Check sheet for the modelled part. Datum: model origin and axes. Units: mm. Face numbers are marked on the shaded views. A direction names the side the tool comes from. Coordinates: 2 decimals unless noted, no trailing zeros. Order: outer loops, then holes, each group sorted by start corner. A loop starts at its lowest first (then second) coordinate and runs counter-clockwise, first axis right, second up.
1. Thickness scan on line 1 (Y direction, x = 10, z = 2.3); line 2 (X direction, y = 20.5, z = 2.9); line 3 (X direction, y = 6.25, z = 2). Record the ranges inside material, lowest first.
2. Cross-section at C-C (x = 10). Enter the section's corners in (y, z) (3 decimals).
3. Set-up check for the marked faces 1 and 2: record each of +Z, -Z, +X, -X, +Y, -Y from which the full face is reachable in a straight line by a thin tool's end or side.
4. Cross-section at A-A (z = 2.8). Enter the section's corners in (x, y), then the cut area to 3 significant figures.
5. Cross-section at B-B (y = 20.5). Enter the section's corners in (x, z) (3 decimals).
6. Draft check along Y on the marked faces 3, 4, 5 and 6. Enter one of: released by +Y, released by -Y, zero draft, split by the parting line, or undercut.
Autodesk Inventor part; units mm, degrees
ref_plane "YZ Plane" through (0, 0, 0) normal (1, 0, 0) x (0, 1, 0)
ref_plane "XZ Plane" through (0, 0, 0) normal (0, 1, 0) x (-1, 0, 0)
ref_plane "XY Plane" through (0, 0, 0) normal (0, 0, 1) x (1, 0, 0)
sketch "Sketch1" plane through (0, 0, 0) normal (0, 0, 1) x (1, 0, 0)
  line L0 (0, 0) -> (20, 0)
  line L1 (20, 0) -> (20, 41)
  line L2 (20, 41) -> (0, 41)
  line L3 (0, 41) -> (0, 0)
  dimension "d0" = 20
  dimension "d1" = 41
extrude "Extrusion1" add sketch "Sketch1" along normal blind 4
sketch "Sketch2" plane through (0, 0, 4) normal (0, 0, 1) x (1, 0, 0)
  line L0 (20, 0) -> (20, 41)
  line L1 (20, 41) -> (0, 41)
  point P0 (0, 0)
  point P1 (10, 20.5)
  dimension "d11" = 10
  dimension "d12" = 20.5
hole "Hole1" at (10, 20.5, 4) direction (0, 0, -1) diameter 11 end through all counterbore diameter 16.4 counterbore depth 2
sketch "Sketch3" plane through (0, 0, 4) normal (0, 0, 1) x (1, 0, 0)
  line L0 (20, 0) -> (20, 41)
  line L1 (20, 41) -> (0, 41)
  point P0 (0, 0)
  point P1 (10, 34.75)
  dimension "d20" = 10
  dimension "d21" = 6.25
hole "Hole2" at (10, 34.75, 4) direction (0, 0, -1) diameter 4 end through all
sketch "Sketch4" plane through (0, 0, 4) normal (0, 0, 1) x (1, 0, 0)
  line L0 (20, 0) -> (20, 41)
  line L1 (0, 0) -> (20, 0)
  point P0 (10, 6.25)
  dimension "d29" = 10
  dimension "d30" = 6.25
hole "Hole3" at (10, 6.25, 4) direction (0, 0, -1) diameter 4 end through all
fillet "Fillet1" radius 6.35 1 edges at (20, 41, 2)
fillet "Fillet2" radius 6.35 1 edges at (0, 41, 2)
fillet "Fillet3" radius 6.35 1 edges at (20, 0, 2)
fillet "Fillet4" radius 6.35 1 edges at (0, 0, 2)
fillet "Fillet5" radius 1.905 8 edges at (10, 41, 0) (1.8599, 39.1401, 0) (0, 20.5, 0) (1.8599, 1.8599, 0) (10, 0, 0) (18.1401, 1.8599, 0) (20, 20.5, 0) (18.1401, 39.1401, 0)
properties part number "sides"
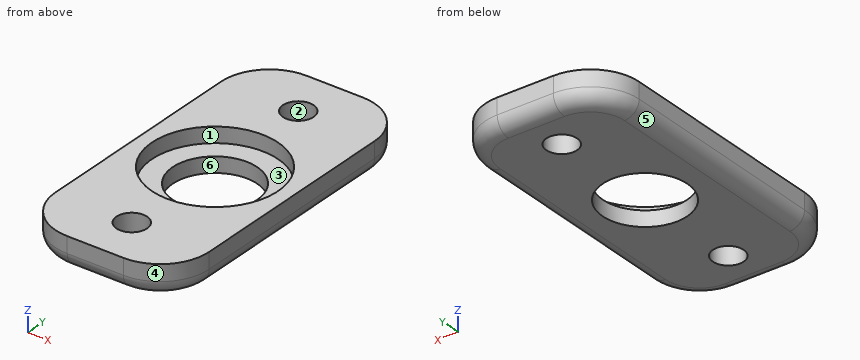
Data:
1. line 1: y = 0 to 4.25, 8.25 to 12.3, 28.7 to 32.75, 36.75 to 41
1. line 2: x = 0 to 1.8, 18.2 to 20
1. line 3: x = 0 to 8, 12 to 20
2. outline: (0, 1.905) arc R1.905 ccw to (1.905, 0) - (4.25, 0) - (4.25, 4) - (0, 4) - close; (8.25, 0) - (15, 0) - (15, 2) - (12.3, 2) - (12.3, 4) - (8.25, 4) - close; (26, 0) - (32.75, 0) - (32.75, 4) - (28.7, 4) - (28.7, 2) - (26, 2) - close; (36.75, 0) - (39.095, 0) arc R1.905 ccw to (41, 1.905) - (41, 4) - (36.75, 4) - close
3. face 1: +Z
3. face 2: +Z, -Z
4. outline: (0, 6.35) arc R6.35 ccw to (6.35, 0) - (13.65, 0) arc R6.35 ccw to (20, 6.35) - (20, 34.65) arc R6.35 ccw to (13.65, 41) - (6.35, 41) arc R6.35 ccw to (0, 34.65) - close; hole circle Ø16.4 at (10, 20.5); hole circle Ø4 at (10, 6.25); hole circle Ø4 at (10, 34.75)
4. area: 549 mm2
5. outline: (0, 1.905) arc R1.905 ccw to (1.905, 0) - (4.5, 0) - (4.5, 2) - (1.8, 2) - (1.8, 4) - (0, 4) - close; (15.5, 0) - (18.095, 0) arc R1.905 ccw to (20, 1.905) - (20, 4) - (18.2, 4) - (18.2, 2) - (15.5, 2) - close
6. face 3: undercut
6. face 4: released by -Y
6. face 5: zero draft
6. face 6: undercut
